from build123d import *

# Parameters (mm, degrees)
SZKIC1_W                    = 28
SZKIC1_H                    = 6
SZKIC1_R                    = 1.65
DODANIE_WYCI_GNI_CIE1_DEPTH = 3
SZKIC2_W                    = 28
SZKIC2_H                    = 3
DODANIE_WYCI_GNI_CIE2_DEPTH = 3
SZKIC3_R                    = 1.65
DODANIE_WYCI_GNI_CIE4_DEPTH = 28
WYTNIJ_WYCI_GNI_CIE2_DEPTH  = 10
SFAZOWANIE1_START           = -14
SFAZOWANIE1_DEPTH           = 28
SFAZOWANIE1_START_2         = -4
SFAZOWANIE1_2_DEPTH         = 8
SZKIC5_W                    = 0.893182681
SZKIC5_H                    = 1.710314622
WYTNIJ_WYCI_GNI_CIE3_DEPTH  = 10
SZKIC6_W                    = 13
SZKIC6_H                    = 3
WYTNIJ_WYCI_GNI_CIE4_DEPTH  = 1.5
DODANIE_WYCI_GNI_CIE5_DEPTH = 6
SZKIC9_R                    = 15
WYTNIJ_WYCI_GNI_CIE5_DEPTH  = 3
SFAZOWANIE2_SIZE            = 4
SFAZOWANIE3_SIZE            = 4
DODANIE_WYCI_GNI_CIE6_DEPTH = 2
SFAZOWANIE4_SIZE            = 1
SFAZOWANIE5_SIZE            = 1
DODANIE_WYCI_GNI_CIE7_DEPTH = 8


with BuildPart() as part:
    # Szkic1 → Dodanie-wyciągnięcie1 (new body)
    with BuildSketch(Plane.XY):
        Rectangle(SZKIC1_W, SZKIC1_H)
        with Locations((11, 0)):
            Circle(SZKIC1_R, mode=Mode.SUBTRACT)
        with Locations((-11, 0)):
            Circle(SZKIC1_R, mode=Mode.SUBTRACT)
    extrude(amount=DODANIE_WYCI_GNI_CIE1_DEPTH)

    # Szkic2 → Dodanie-wyciągnięcie2 (add)
    with BuildSketch(Plane.XZ.offset(3)):
        with Locations((0, 1.5)):
            Rectangle(SZKIC2_W, SZKIC2_H)
    extrude(amount=DODANIE_WYCI_GNI_CIE2_DEPTH)

    # Szkic3 → Dodanie-wyciągnięcie4 (add)
    with BuildSketch(Plane(origin=(14, 0, 0), x_dir=(0, 0, -1), z_dir=(1, 0, 0))):
        with BuildLine():
            Line((0, -4.65), (-3, -4.65))
            Line((-3, -4.65), (-3, -7.65))
            ThreePointArc((-3, -7.65), (2.121320344, -9.771320344), (0, -4.65))
        make_face()
        with Locations(Location((0, -7.65, 0), (0, 0, 90))):
            Circle(SZKIC3_R, mode=Mode.SUBTRACT)
    extrude(amount=-DODANIE_WYCI_GNI_CIE4_DEPTH)

    # Szkic4 → Wytnij-wyciągnięcie2 (cut)
    with BuildSketch(Plane.ZY.offset(14)):
        Polygon((-3.162330393, -4.65), (-3.162330393, -3.615751975), (3, -3.615751975), (3, -4.65), (3, -10.796501094), (-3.162330393, -10.796501094), align=None)
    wytnij_wyci_gni_cie2 = extrude(amount=-WYTNIJ_WYCI_GNI_CIE2_DEPTH, mode=Mode.SUBTRACT)

    # Lustro1: Wytnij-wyciągnięcie2 across plane
    add(wytnij_wyci_gni_cie2.mirror(Plane(origin=(0, 0, 0), x_dir=(0, 0, 1), z_dir=(1, 0, 0))), mode=Mode.SUBTRACT)

    # Sfazowanie1: read off the stored shape, not the designer's step
    # Sfazowanie1 outline → Sfazowanie1 (add)
    with BuildSketch(Plane.YZ.offset(SFAZOWANIE1_START)):
        Polygon((-3.615751975, 0), (-3.615751975, -0.893182681), (-1.905437353, 0), align=None)
    extrude(amount=SFAZOWANIE1_DEPTH)

    # Sfazowanie1 2 outline → Sfazowanie1 2 (add)
    with BuildSketch(Plane.YZ.offset(SFAZOWANIE1_START_2)):
        with BuildLine():
            Line((-5.18804458, -1.714285714), (-3.615751975, -0.893182681))
            Line((-3.615751975, -0.893182681), (-3.615751975, 0))
            Line((-3.615751975, 0), (-4.65, 0))
            ThreePointArc((-4.65, 0), (-4.787669982, -0.898369005), (-5.18804458, -1.714285714))
        make_face()
    extrude(amount=SFAZOWANIE1_2_DEPTH)

    # Szkic5 → Wytnij-wyciągnięcie3 (cut)
    with BuildSketch(Plane(origin=(14, 0, 0), x_dir=(0, 0, -1), z_dir=(1, 0, 0))):
        with Locations((0.446591341, -2.760594664)):
            Rectangle(SZKIC5_W, SZKIC5_H)
    wytnij_wyci_gni_cie3 = extrude(amount=-WYTNIJ_WYCI_GNI_CIE3_DEPTH, mode=Mode.SUBTRACT)

    # Lustro2: Wytnij-wyciągnięcie3 across plane
    add(wytnij_wyci_gni_cie3.mirror(Plane(origin=(0, 0, 0), x_dir=(0, 0, 1), z_dir=(1, 0, 0))), mode=Mode.SUBTRACT)

    # Szkic6 → Wytnij-wyciągnięcie4 (cut)
    with BuildSketch(Plane.XY.offset(3)):
        Rectangle(SZKIC6_W, SZKIC6_H)
    extrude(amount=-WYTNIJ_WYCI_GNI_CIE4_DEPTH, mode=Mode.SUBTRACT)

    # Szkic8 → Dodanie-wyciągnięcie5 (add)
    with BuildSketch(Plane.ZY.offset(14)):
        with BuildLine():
            Line((3, 3), (3, 7.046938457))
            ThreePointArc((3, 7.046938457), (-15, -7.65), (3, -22.346938457))
            Line((3, -22.346938457), (3, -18.3))
            ThreePointArc((3, -18.3), (-10.65, -10.65), (-3, 3))
            Line((-3, 3), (0, 3))
            Line((0, 3), (3, 3))
        make_face()
    extrude(amount=-DODANIE_WYCI_GNI_CIE5_DEPTH)

    # Szkic9 → Wytnij-wyciągnięcie5 (cut)
    with BuildSketch(Plane.ZY.offset(14)):
        with Locations((0, -7.65)):
            Circle(SZKIC9_R)
        with BuildLine():
            Line((-3, 3), (3, 3))
            ThreePointArc((3, 3), (0, -18.714470164), (-3, 3))
        make_face(mode=Mode.SUBTRACT)
    extrude(amount=-WYTNIJ_WYCI_GNI_CIE5_DEPTH, mode=Mode.SUBTRACT)

    # Sfazowanie2
    sfazowanie2_edges = [part.edges().sort_by_distance(p)[0] for p in [
        (-8, 3, 1.5),
    ]]
    chamfer(sfazowanie2_edges, length=SFAZOWANIE2_SIZE)

    # Sfazowanie3
    # the kernel refuses this chamfer: 4 mm, written as the material it adds along each edge
    with BuildSketch(Plane(origin=(-11, 3, 0), x_dir=(-1, 0, 0), z_dir=(0, 0, 1))) as sfazowanie3_piece_1_section:
        Polygon((SFAZOWANIE3_SIZE, 0), (0, -SFAZOWANIE3_SIZE), (0, 0), align=None)
    sfazowanie3_piece_1 = extrude(amount=3, mode=Mode.PRIVATE)
    sfazowanie3_piece_1 = split(sfazowanie3_piece_1, bisect_by=Plane(origin=(-14, 3, 0), z_dir=(1, 0, 0)), keep=Keep.TOP, mode=Mode.PRIVATE)
    add(sfazowanie3_piece_1)

    # Szkic10 → Dodanie-wyciągnięcie6 (add)
    with BuildSketch(Plane(origin=(0, 0, 0), x_dir=(-1, 0, 0), z_dir=(0, 0, -1))):
        Polygon((-8, 3), (-8, -3.615751975), (8, -3.615751975), (8, 3.615751975), (8, 7), (4, 3), align=None)
    extrude(amount=DODANIE_WYCI_GNI_CIE6_DEPTH)

    # Sfazowanie4
    sfazowanie4_edges = [part.edges().sort_by_distance(p)[0] for p in [
        (-8, 5, -2),
    ]]
    chamfer(sfazowanie4_edges, length=SFAZOWANIE4_SIZE)

    # Sfazowanie5
    sfazowanie5_edges = [part.edges().sort_by_distance(p)[0] for p in [
        (-11, 5, 0),
    ]]
    chamfer(sfazowanie5_edges, length=SFAZOWANIE5_SIZE)

    # Szkic11 → Dodanie-wyciągnięcie7 (add)
    with BuildSketch(Plane(origin=(4, 0, 0), x_dir=(0, 0, -1), z_dir=(1, 0, 0))):
        Polygon((2, -3.615751975), (2, -5.632292806), (0.35679852, -3.615751975), align=None)
    extrude(amount=-DODANIE_WYCI_GNI_CIE7_DEPTH)


solid = part.part
Model file for the job. Use its own axes, mm. A direction names the side the tool comes from. Give positions to 0.01 mm unless a question says otherwise; leave off trailing zeros. Write each loop counter-clockwise with the first axis right and the second up, starting at its lowest first coordinate (ties: lowest second). Pieces come first, ordered by that corner, then holes. Notation, with made-up numbers: M 50,30 L 68,30 A25 ccw 68,58 Z; hole C 84,47 d4. An arc over 180 degrees is marked long. One line per item, written item: value. Start each with the question number.
Q1. Drop flat-ended pins along their axis: pin 1 Ø2.5 at (x, z) = (-10, -1.5) entering from -Y; pin 2 Ø1.8 at (x, y) = (10.5, -1) entering from -Z; pin 3 Ø2 at (y, z) = (-9, -8) entering from -X; pin 4 Ø1.8 at (y, z) = (-7, 1) entering from -X. Give the stop position or say it passes through.
Q2. Saw through at A-A, the plane x = 11. Write the cut outline in (y, z), plus the area to 3 significant figures.
Q3. Saw through at C-C, the plane x = 3. Write the cut outline in (y, z), plus the area to 3 significant figures.
Q4. Two-plate mould, pull along Z, no slides. Class faces 6 (the flat face through (-11.5, 4.6, -0.5)), 7 (the flat face through (-8, 0, -1)), 8 (the flat face through (-4, -6, 1)), 9 (the flat face through (0, 0, 1.5)): +Z half, -Z half, draft (parallel to the pull), parting line (faces both ways), or undercut.
Q5. 3-axis set-ups, long thin cutter, end or side, ignore diameter. For faces 1 (the flat face through (4, -6, 1)), 2 (the flat face through (11, -2, 0)), 3 (the flat face through (-10, 3, -2)), 4 (the flat face through (0, 1.5, 2)), 5 (the flat face through (3, 3, 1)): which of +Z, -Z, +X, -X, +Y, -Y reach the whole face in a straight line?
Q6. Saw through at D-D, the plane x = -5.5. Write the cut outline in (y, z).
Q7. Saw through at B-B, the plane z = -3.5. Write the cut outline in (x, y), plus the area to 3 significant figures.
Q8. Probe probe 1 along Y at (x, z) = (11, 1.95); probe 2 along X at (y, z) = (-14, -10.75); probe 3 along Z at (x, y) = (0.5, -7.65). List the from-to ranges inside material, lowest first. Write a range as [from, to].
Output values:
1. pin 1: stops at y = -22.65
1. pin 2: stops at z = 0
1. pin 3: passes through
1. pin 4: stops at x = -4
2. outline: M -3.62,0 L -1.65,0 L -1.65,3 L -3.62,3 Z; M 1.65,0 L 3,0 L 3,3 L 1.65,3 Z
2. area: 9.95 mm²
3. outline: M -7.65,3 A3 ccw long -5.41,-2 L 3,-2 L 3,3 L 1.5,3 L 1.5,1.5 L -1.5,1.5 L -1.5,3 Z; hole C -7.65,0 d3.3
3. area: 55.9 mm²
4. face 6: -Z half
4. face 7: undercut
4. face 8: draft
4. face 9: +Z half
5. face 1: +Z, -Z, +X, -Y
5. face 2: -Z, +X, +Y, -Y
5. face 3: -X
5. face 4: +Z
5. face 5: +Z, -Z, +X, +Y
6. outline: M -3.62,-2 L 4.5,-2 L 4.5,3 L 1.5,3 L 1.5,1.5 L -1.5,1.5 L -1.5,3 L -3.62,3 Z
7. outline: M -11,-22.24 L -8,-22.24 L -8,-18.15 L -11,-18.15 Z; M -11,2.85 L -8,2.85 L -8,6.94 L -11,6.94 Z
7. area: 24.5 mm²
8. probe 1: y = [-3.62, -1.65], [1.65, 3]
8. probe 2: x = [-11, -8]
8. probe 3: z = [-3, -1.65], [1.65, 3]
